The listing builds one solid part. Answer for the finished solid, in the listing's coordinates (mm). A direction names the side the tool comes from. Round coordinates to 2 decimals unless told otherwise and drop trailing zeros. Loops run counter-clockwise (first coordinate to the right, second up) from the corner with the lowest first, then second, coordinate; pieces in that order, holes last. Notation, with made-up numbers: (86.25, 9) -> (122.25, 9) arc R14 cw to (122.25, 32) -> close; hole circle Ø6 at (45, 87). An arc over 180 degrees is marked (long way). Use a Markdown table: item, result. Add a question column.
Q1. Section A-A on y = -12.5 is taken. Give the vertices of the cut face in (x, z).
Q2. Section B-B on y = 19.5 is taken. Give the vertices of the cut face in (x, z), then the cut area to 3 significant figures.
Q3. Given pin 1 Ø8 at (x, y) = (3.5, 16) entering from +Z; pin 2 Ø8 at (y, z) = (-10.5, 25) entering from +X; pin 3 Ø12 at (y, z) = (-38.5, -1) entering from -X; pin 4 Ø24 at (x, z) = (3, 2) entering from -Y, each flat-ended and moving along its own axis, determine where each tip first touches the part or whether it passes through.
Q4. For a pull along Z with two mould halves and no side action, classify faces 1 (the flat face through (0, 0, 0)), 2 (the conical face through (-5.914, 22.044, 4.535)), 3 (the flat face through (-10, -75.047, 10)) as released by +Z, released by -Z, zero draft, split by the parting line, or undercut.
Q5. Consider line 1 (Z direction, x = 0, y = -23); line 2 (Y direction, x = -16, z = -37.5). Determine where each line is inside the solid, lowest interval first.
Q6. Section C-C on y = -31.5 is taken. Give the vertices of the cut face in (x, z), then the cut area to 3 significant figures.
Q7. Which of the six approach directions +Z, -Z, +X, -X, +Y, -Y give full straight-line access (tool end or side, diameter ignored) to faces 4 (the cylindrical face through (10.418, -36.998, 3.281)), 5 (the cylindrical face through (-3.58, -13.42, -27.29)), 6 (the conical face through (-22.57, -55.59, 17.31))?
from build123d import *

# Parameters (mm, degrees)
F2_R     = 10.922
F3_DEPTH = 429.26


with BuildPart() as f1:
    # F0 (on Top) → F1 (revolve)
    with BuildSketch(Plane.XY):
        Polygon((0, -75.046971), (46.471976, -75.046971), (27.522236, -54.593291), (45.268815, -51.585395), (27.522236, -27.221449), (27.522236, 0), (0, 30.229341), align=None)
    revolve(axis=Axis((0, -22.408815, 0), (0, 1, 0)))

    # F2 (on Front) → F3 (cut)
    with BuildSketch(Plane.XZ):
        Circle(F2_R)
    extrude(amount=F3_DEPTH, mode=Mode.SUBTRACT)


solid = f1.part
Checked values:
| question | item | result |
|---|---|---|
| 1 | outline | circle Ø55.04 at (0, 0); hole circle Ø21.84 at (0, 0) |
| 2 | outline | circle Ø19.54 at (0, 0) |
| 2 | area | 300 mm2 |
| 3 | pin 1 | stops at z = 16.3 |
| 3 | pin 2 | stops at x = 17.79 |
| 3 | pin 3 | stops at x = -40.1 |
| 3 | pin 4 | stops at y = -75.05 |
| 4 | face 1 | undercut |
| 4 | face 2 | split by the parting line |
| 4 | face 3 | zero draft |
| 5 | line 1 | z = -27.52 to -10.92, 10.92 to 27.52 |
| 5 | line 2 | y = -75.05 to -68.89, -52.35 to -45.41 |
| 6 | outline | circle Ø61.28 at (0, 0); hole circle Ø21.84 at (0, 0) |
| 6 | area | 2,570 mm2 |
| 7 | face 4 | -Y |
| 7 | face 5 | +Y |
| 7 | face 6 | none |
